from build123d import *

# Parameters (mm, degrees)
SKETCH2_R           = 5
BOSS_EXTRUDE2_DEPTH = 20


with BuildPart() as part:
    # Sketch2 → Boss-Extrude2 (new body)
    with BuildSketch(Plane.XY):
        with BuildLine():
            ThreePointArc((-49, -9.949874371), (-43.301270189, -25), (-33.11684397, -37.4603076))
            ThreePointArc((-33.11684397, -37.4603076), (-30, -51.961524227), (-15.88315603, -47.410181971))
            ThreePointArc((-15.88315603, -47.410181971), (0, -50), (15.88315603, -47.410181971))
            ThreePointArc((15.88315603, -47.410181971), (30, -51.961524227), (33.11684397, -37.4603076))
            ThreePointArc((33.11684397, -37.4603076), (43.301270189, -25), (49, -9.949874371))
            ThreePointArc((49, -9.949874371), (60, 0), (49, 9.949874371))
            ThreePointArc((49, 9.949874371), (43.301270189, 25), (33.11684397, 37.4603076))
            ThreePointArc((33.11684397, 37.4603076), (30, 51.961524227), (15.88315603, 47.410181971))
            ThreePointArc((15.88315603, 47.410181971), (0, 50), (-15.88315603, 47.410181971))
            ThreePointArc((-15.88315603, 47.410181971), (-30, 51.961524227), (-33.11684397, 37.4603076))
            ThreePointArc((-33.11684397, 37.4603076), (-43.301270189, 25), (-49, 9.949874371))
            ThreePointArc((-49, 9.949874371), (-60, 0), (-49, -9.949874371))
        make_face()
        with Locations((-50, 0)):
            Circle(SKETCH2_R, mode=Mode.SUBTRACT)
        with Locations((-25, 43.301270189)):
            Circle(SKETCH2_R, mode=Mode.SUBTRACT)
        with Locations((25, 43.301270189)):
            Circle(SKETCH2_R, mode=Mode.SUBTRACT)
        with Locations((50, 0)):
            Circle(SKETCH2_R, mode=Mode.SUBTRACT)
        with Locations((25, -43.301270189)):
            Circle(SKETCH2_R, mode=Mode.SUBTRACT)
        with Locations((-25, -43.301270189)):
            Circle(SKETCH2_R, mode=Mode.SUBTRACT)
        with BuildLine():
            ThreePointArc((34.641016151, 20), (24.35045716, 31.734133612), (10.352761804, 38.637033052))
            ThreePointArc((10.352761804, 38.637033052), (4.229037447, 35.101499146), (7.764571353, 28.977774789))
            ThreePointArc((7.764571353, 28.977774789), (18.26284287, 23.800600209), (25.980762114, 15))
            ThreePointArc((25.980762114, 15), (32.810889132, 13.169872981), (34.641016151, 20))
        make_face(mode=Mode.SUBTRACT)
        with BuildLine():
            ThreePointArc((0, -40), (15.307337295, -36.9551813), (28.284271247, -28.284271247))
            ThreePointArc((28.284271247, -28.284271247), (28.284271247, -21.213203436), (21.213203436, -21.213203436))
            ThreePointArc((21.213203436, -21.213203436), (11.480502971, -27.716385975), (0, -30))
            ThreePointArc((0, -30), (-5, -35), (0, -40))
        make_face(mode=Mode.SUBTRACT)
        with BuildLine():
            ThreePointArc((-34.641016151, 20), (-39.657794455, 5.221047689), (-38.637033052, -10.352761804))
            ThreePointArc((-38.637033052, -10.352761804), (-32.513308695, -13.88829571), (-28.977774789, -7.764571353))
            ThreePointArc((-28.977774789, -7.764571353), (-29.743345841, 3.915785767), (-25.980762114, 15))
            ThreePointArc((-25.980762114, 15), (-27.810889132, 21.830127019), (-34.641016151, 20))
        make_face(mode=Mode.SUBTRACT)
    extrude(amount=BOSS_EXTRUDE2_DEPTH)


solid = part.part
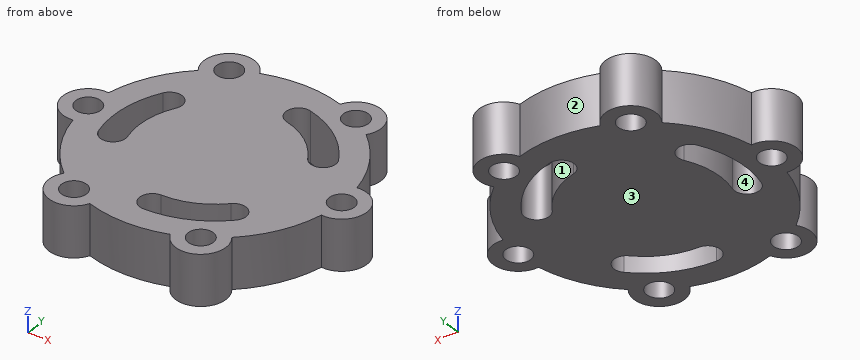
Could you check a few things on this model? Use its own coordinates, in mm. Face numbers are marked on the shaded views. A direction names the side the tool comes from. Give positions to 0.01 mm unless a question says otherwise; leave off trailing zeros. Order: outer loops, then holes, each group sorted by start corner. A loop starts at its lowest first (then second) coordinate and runs counter-clockwise, first axis right, second up.
1. We'd pull the mould along X, two halves only. Please class the marked faces 3 and 4: pulls with the +X half, pulls with the -X half, needs draft (parallel to the pull), parting line crosses it, or undercut.
2. Suppose I cut it at D-D (y = -35). List the corners of the cut face in (x, z) for me.
3. For the marked faces 1 and 2, which set-ups out of +Z, -Z, +X, -X, +Y, -Y let a thin tool reach every point of the face, with its end or its side?
4. Suppose I cut it at C-C (z = 15.75). Give the number of separate pieces and of enclosed holes in the cut face, plus the area to 3 significant figures.
5. Suppose I cut it at A-A (y = 0). List the corners of the cut face in (x, z) for me, plus the area to 3 significant figures.
6. Suppose I cut it at B-B (x = -23.5). List the corners of the cut face in (y, z) for me.
7. I need wall thicknesses on L1, parallel to Y at x = -25, z = 13.25; L2, parallel to X at y = 39, z = 1.75; L3, parallel to X at y = 21, z = 2.75. Which ranges of each line are inside material? Lowest first, please.
8. Will these pins go through, and if not, where does the flat tip stop? P1, Ø6, axis at x = 46.5, z = 12, coming from the +Y side; P2, Ø5, axis at x = -28.5, z = 18, coming from the +Y side; P3, Ø6, axis at x = 44.5, z = 3, coming from the +Y side; P4, Ø8, axis at x = -50, y = 0, coming from the +Z side.
Solved:
1. face 3: needs draft
1. face 4: undercut
2. outline: (-35.71, 0) - (-5, 0) - (-5, 20) - (-35.71, 20) - close; (19.36, 0) - (35.71, 0) - (35.71, 20) - (19.36, 20) - close
3. face 1: +Z, -Z
3. face 2: +Z, -Z, +Y
4. separate pieces: 1
4. enclosed holes: 9
4. area: 7,300 mm2
5. outline: (-60, 0) - (-55, 0) - (-55, 20) - (-60, 20) - close; (-45, 0) - (-40, 0) - (-40, 20) - (-45, 20) - close; (-30, 0) - (45, 0) - (45, 20) - (-30, 20) - close; (55, 0) - (60, 0) - (60, 20) - (55, 20) - close
5. area: 1,800 mm2
6. outline: (-53.19, 0) - (-48.07, 0) - (-48.07, 20) - (-53.19, 20) - close; (-38.53, 0) - (38.53, 0) - (38.53, 20) - (-38.53, 20) - close; (48.07, 0) - (53.19, 0) - (53.19, 20) - (48.07, 20) - close
7. L1: y = -53.3 to -48.3, -38.3 to 38.3, 48.3 to 53.3
7. L2: x = -34.03 to -27.55, -22.45 to 22.45, 27.55 to 34.03
7. L3: x = -45.38 to -33.88, -26.74 to 21.42, 34.04 to 45.38
8. P1: stops at y = 24.65
8. P2: stops at y = 53.25
8. P3: stops at y = 27.89
8. P4: passes through
